```python
from build123d import *

# Parameters (mm, degrees)
F1_DEPTH = 6.35
F2_R     = 5.08
F3_R     = 5.08


with BuildPart() as f1:
    # F0 (on Front) → F1 (new body)
    with BuildSketch(Plane.XZ):
        with BuildLine():
            ThreePointArc((0, -55.016398), (16.101153, -27.176721), (46.024799, -15.3924))
            ThreePointArc((46.024799, -15.3924), (55.101189, -4.894395), (68.087099, 0))
            Line((68.087099, 0), (36.271196, 0))
            ThreePointArc((36.271196, 0), (23.424104, -5.290842), (9.753601, -7.772401))
            Line((9.753601, -7.772401), (9.753601, 4.927599))
            Line((9.753601, 4.927599), (6.4008, 0))
            ThreePointArc((6.4008, 0), (0, 2.593731), (-6.4008, 0))
            Line((-6.4008, 0), (-9.753601, 4.927599))
            Line((-9.753601, 4.927599), (-9.753601, -7.772401))
            ThreePointArc((-9.753601, -7.772401), (-23.424104, -5.290842), (-36.271196, 0))
            Line((-36.271196, 0), (-68.087099, 0))
            ThreePointArc((-68.087099, 0), (-55.101189, -4.894395), (-46.024799, -15.3924))
            ThreePointArc((-46.024799, -15.3924), (-16.101153, -27.176721), (0, -55.016398))
        make_face()
    extrude(amount=F1_DEPTH)

    # F2
    f2_edges = [f1.edges().sort_by_distance(p)[0] for p in [
        (-55.101189, -6.35, -4.894395),
    ]]
    fillet(f2_edges, radius=F2_R)

    # F3
    f3_edges = [f1.edges().sort_by_distance(p)[0] for p in [
        (55.101189, -6.35, -4.894395),
    ]]
    fillet(f3_edges, radius=F3_R)


solid = f1.part
```
Design review of the part built by this model. Coordinates are the model's own, in mm. A direction names the side the tool comes from. Give positions to 0.01 mm unless a question says otherwise; leave off trailing zeros. Write each loop counter-clockwise with the first axis right and the second up, starting at its lowest first coordinate (ties: lowest second). Pieces come first, ordered by that corner, then holes.
(1) Wall thickness on line 1 along X through (y, z) = (-4.25, -3); line 2 along Z through (x, y) = (-25, -2.75); line 3 along X through (y, z) = (-2, -38): over which ranges is each line inside the solid? List them lowest first.
Checked values:
line 1: x = -56.25 to -29.95, -9.75 to 9.75, 29.95 to 56.25
line 2: z = -21.09 to -4.81
line 3: x = -6.74 to 6.74
(2) Add section B-B (z = -26). Give the boundary of the cut face in (x, y).
Checked values:
outline: (-17.52, -6.35) - (17.52, -6.35) - (17.52, 0) - (-17.52, 0) - close
(3) Clearance check with flat-ended pins moving along their axes: pin 1 Ø3 at (x, y) = (51, -2) entering from +Z; pin 2 Ø1 at (x, y) = (-32, -5) entering from +Z. State where each tip first meets the part, or that it passes through.
Checked values:
pin 1: stops at z = 0
pin 2: stops at z = -1.89
(4) Add section A-A (y = -5). Give the boundary of the cut face in (x, z), and give its area (3 significant figures).
Checked values:
outline: (-61.01, 0) arc R29.82 cw to (-44.16, -15.5) arc R48.82 cw to (0, -55.02) arc R48.82 cw to (44.16, -15.5) arc R29.82 cw to (61.01, 0) - (36.27, 0) arc R65.94 cw to (9.75, -7.77) - (9.75, 4.93) - (6.4, 0) arc R9.19 ccw to (-6.4, 0) - (-9.75, 4.93) - (-9.75, -7.77) arc R65.94 cw to (-36.27, 0) - close
area: 2,270 mm2
(5) Mouldability with a two-part tool opening along X and no side actions: class faces 6 (the face through (15.75, -3.13, -27.48)), 7 (the face through (0.099, -3.131, 2.593)), 8 (the face through (-16.45, -3.13, -26.88)), 9 (the face through (0, 0, -14)) as +X half, -X half, draft (parallel to the pull), parting line (faces both ways), or undercut.
Checked values:
face 6: +X half
face 7: undercut
face 8: -X half
face 9: draft
(6) Add section C-C (x = 20.5). Give the boundary of the cut face in (y, z), and give its area (3 significant figures).
Checked values:
outline: (-6.35, -23.8) - (0, -23.8) - (0, -6.08) - (-6.35, -6.08) - close
area: 113 mm2
(7) Tool access review of faces 1 (the face through (-52, -3, 0)), 2 (the face through (-9.754, -3, -1)), 3 (the face through (54.94, -0.63, -5.01)), 4 (the face through (52, -3, 0)), 5 (the face through (-55.263, -0.626, -4.783)): name each direction out of +Z, -Z, +X, -X, +Y, -Y from which nothing blocks a thin tool from reaching the whole face with its end or side.
Checked values:
face 1: +Z, -X, +Y, -Y
face 2: +Z, +Y, -Y
face 3: -Z, +X, +Y, -Y
face 4: +Z, +X, +Y, -Y
face 5: -Z, -X, +Y, -Y
